from build123d import *

# Parameters (mm, degrees)
F0_W     = 63.5
F0_H     = 63.5
F1_DEPTH = 63.5
F2_W     = 63.5
F2_H     = 63.5
F2_R     = 19.171796
F3_DEPTH = 25.4
F4_R     = 12.7
F5_DEPTH = 63.754


with BuildPart() as f1:
    # F0 (on Front) → F1 (new body)
    with BuildSketch(Plane.XZ):
        with Locations((4.171845, -1.547694)):
            Rectangle(F0_W, F0_H)
    extrude(amount=F1_DEPTH)

    # F2 (on face) → F3 (cut)
    with BuildSketch(Plane.XZ.offset(63.5)):
        with Locations((4.171845, -1.547694)):
            Rectangle(F2_W, F2_H)
        with Locations((4.171845, -1.547694)):
            Circle(F2_R, mode=Mode.SUBTRACT)
    extrude(amount=-F3_DEPTH, mode=Mode.SUBTRACT)

    # F4 (on face) → F5 (cut)
    with BuildSketch(Plane.XZ.offset(63.5)):
        with Locations((4.171845, -1.547694)):
            Circle(F4_R)
    extrude(amount=-F5_DEPTH, mode=Mode.SUBTRACT)


solid = f1.part
Geometry: final body of the model. Coordinates: model frame, mm. A direction names the side the tool comes from. Give positions to 0.01 mm unless a question says otherwise; leave off trailing zeros. Loops run counter-clockwise (first coordinate to the right, second up) from the corner with the lowest first, then second, coordinate; pieces in that order, holes last. Notation, with made-up numbers: M 51.25,56 L 97.25,56 A23 cw 97.25,65 Z; hole C 7,87 d1. An arc over 180 degrees is marked long. Put each result on its own line as item: value. Start each with the question number.
1) Cut plane D-D (z = -19). Output: boundary loops of the cut face in (x, y), then the cut area to 3 significant figures.
2) Ray query, line 1 along X through (y, z) = (-21, -2); line 2 along X through (y, z) = (-47, 7); line 3 along Z through (x, y) = (-3, -21). Return the intervals inside material, ascending.
3) Contact query for flat-ended pins moving along their axis: pin 1 (1 mm diameter, centred on x = -12.5, z = 9, fed in from -Y); pin 2 (6 mm diameter, centred on x = 2.5, y = -57, fed in from +Z); pin 3 (1 mm diameter, centred on x = 0, y = -51.5, fed in from -Z). Output: stop coordinate, or through.
4) Cut plane A-A (x = 9). Output: boundary loops of the cut face in (y, z).
5) Cut plane C-C (z = -6.5). Output: boundary loops of the cut face in (x, y).
6) Cut plane B-B (y = -7). Output: boundary loops of the cut face in (x, z), then the cut area to 3 significant figures.
7) Pull-direction query (Z, two-part tool) for faces 1 (the flat face through (35.922, -19, -2)), 2 (the cylindrical face through (1.419, -32.194, -13.946)), 3 (the flat face through (4, -19, 30.202)), 4 (the flat face through (4, -19, -33.298)); classes: pulls with the +Z half, pulls with the -Z half, needs draft (parallel to the pull), parting line crosses it, or undercut.
8) Access query for faces 5 (the flat face through (17, -63.5, -6)), 6 (the cylindrical face through (22.46, -50.98, 4.21)). Directions: +Z, -Z, +X, -X, +Y, -Y. A direction counts if a zero-diameter tool reaches every point of the face in a straight line with its end or side. Return the directions, or none.
Verdict:
1. outline: M -27.58,-38.1 L -3.76,-38.1 L -3.76,-63.5 L 12.11,-63.5 L 12.11,-38.1 L 35.92,-38.1 L 35.92,0 L -27.58,0 Z
1. area: 2,820 mm2
2. line 1: -27.58 to -8.52, 16.86 to 35.92
2. line 2: -12.99 to -5.22, 13.56 to 21.33
2. line 3: -33.3 to -12.03, 8.93 to 30.2
3. pin 1: y = -38.1
3. pin 2: z = 17.62
3. pin 3: z = -20.36
4. outline: M -63.5,-20.1 L -38.1,-20.1 L -38.1,-33.3 L 0,-33.3 L 0,-13.29 L -63.5,-13.29 Z; M -63.5,10.2 L 0,10.2 L 0,30.2 L -38.1,30.2 L -38.1,17.01 L -63.5,17.01 Z
5. outline: M -27.58,-38.1 L -14.35,-38.1 L -14.35,-63.5 L -7.52,-63.5 L -7.52,0 L -27.58,0 Z; M 15.87,-63.5 L 22.69,-63.5 L 22.69,-38.1 L 35.92,-38.1 L 35.92,0 L 15.87,0 Z
6. outline: M -27.58,-33.3 L 35.92,-33.3 L 35.92,30.2 L -27.58,30.2 Z; hole C 4.17,-1.55 d25.4
6. area: 3,530 mm2
7. face 1: needs draft
7. face 2: undercut
7. face 3: pulls with the +Z half
7. face 4: pulls with the -Z half
8. face 5: +Z, -Z, +X, -X, -Y
8. face 6: -Y
